Can you work these out from the model? Positions are in its coordinate system, mm. Round coordinates to 2 decimals unless told otherwise and drop trailing zeros. Write each loop counter-clockwise with the first axis right and the second up, starting at its lowest first coordinate (ties: lowest second). Pieces come first, ordered by that corner, then holes. Notation, with made-up numbers: M 79.5,64 L 87.5,64 A17 cw 87.5,96 Z; hole C 76.5,75.5 d9. An arc over 180 degrees is marked long. Answer in a Markdown table with one row per item. Add a question column.
(1) I'm going to push flat-ended pins straight in: pin 1 (3 mm diameter, centred on x = 1187, z = -6, fed in from -Y); pin 2 (2 mm diameter, centred on x = 1224.5, z = -2.5, fed in from +Y); pin 3 (1.5 mm diameter, centred on x = 1410.5, y = -968.5, fed in from +Z); pin 4 (3 mm diameter, centred on y = -743, z = -8.5, fed in from +X). Where does each tip first touch, or does it pass through?
(2) Suppose I cut it at A-A, the plane z = -2. Write out the boundary of the cut face in (x, y), then the cut area to 3 significant figures.
(3) Suppose I cut it at B-B, the plane x = 1329.5. Write out the boundary of the cut face in (y, z), then the cut area to 3 significant figures.
(4) Suppose I cut it at C-C, the plane y = -1021. Write out the boundary of the cut face in (x, z).
(5) If I drill on probe 1 along X at (y, z) = (-1167, -8.5); probe 2 along Y at (x, z) = (1353, -6.75); probe 3 along Y at (x, z) = (1383, -9), over which ranges is the centre line in solid material (lowest first)?
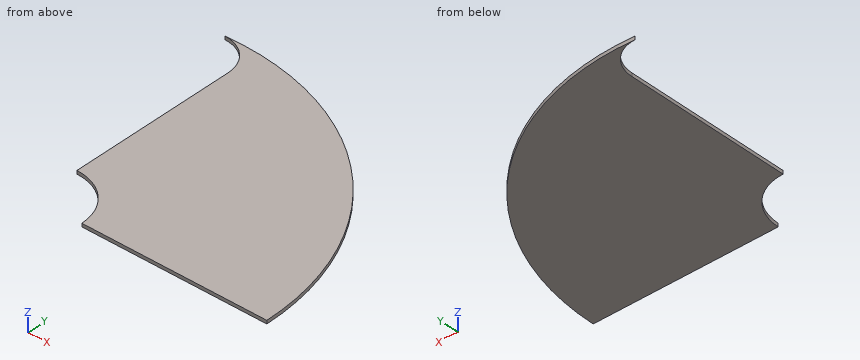
from build123d import *

# Parameters (mm, degrees)
BOSS_EXTRUDE2_DEPTH = 10


with BuildPart() as part:
    # Sketch1 → Boss-Extrude2 (new body)
    with BuildSketch(Plane.XY):
        with BuildLine():
            Line((946.568769473, -612.108653834), (946.568769473, -1116.807153033))
            ThreePointArc((946.568769473, -1116.807153033), (1048.115870255, -1158.869339396), (1090.178056619, -1260.416440178))
            Line((1090.178056619, -1260.416440178), (1646.568769473, -1262.242939545))
            ThreePointArc((1646.568769473, -1262.242939545), (1409.039966295, -713.90421061), (846.568769473, -512.108653834))
            ThreePointArc((846.568769473, -512.108653834), (917.279447592, -541.397975715), (946.568769473, -612.108653834))
        make_face()
    extrude(amount=-BOSS_EXTRUDE2_DEPTH)


solid = part.part
Calculated:
| question | item | result |
|---|---|---|
| 1 | pin 1 | y = -1260.74 |
| 1 | pin 2 | y = -586.19 |
| 1 | pin 3 | z = 0 |
| 1 | pin 4 | x = 1439.84 |
| 2 | outline | M 846.57,-512.11 A100 cw 946.57,-612.11 L 946.57,-1116.81 A143.61 cw 1090.18,-1260.42 L 1646.57,-1262.24 A751.69 ccw Z |
| 2 | area | 390,000 mm² |
| 3 | outline | M -1261.2,-10 L -648.94,-10 L -648.94,0 L -1261.2,0 Z |
| 3 | area | 6,120 mm² |
| 4 | outline | M 946.57,-10 L 1606.81,-10 L 1606.81,0 L 946.57,0 Z |
| 5 | probe 1 | 1055.64 to 1640.51 |
| 5 | probe 2 | -1261.28 to -666.29 |
| 5 | probe 3 | -1261.38 to -690.6 |
